from build123d import *

# Parameters (mm, degrees)
F0_R     = 11
F1_DEPTH = 3
F3_DEPTH = 5


with BuildPart() as f1:
    # F0 (on Top) → F1 (new body)
    with BuildSketch(Plane.XY):
        Circle(F0_R)
    extrude(amount=F1_DEPTH)

    # F2 (on face) → F3 (join)
    with BuildSketch(Plane.XY.offset(3)):
        with BuildLine():
            Line((6, 2.5), (6, 4.5))
            ThreePointArc((6, 4.5), (0, 7.5), (-6, 4.5))
            Line((-6, 4.5), (-6, 2.5))
            ThreePointArc((-6, 2.5), (0, 6.5), (6, 2.5))
        make_face()
        with BuildLine():
            Line((6, -4.5), (6, -2.5))
            ThreePointArc((6, -2.5), (0, -6.5), (-6, -2.5))
            Line((-6, -2.5), (-6, -4.5))
            ThreePointArc((-6, -4.5), (0, -7.5), (6, -4.5))
        make_face()
    extrude(amount=F3_DEPTH)


solid = f1.part
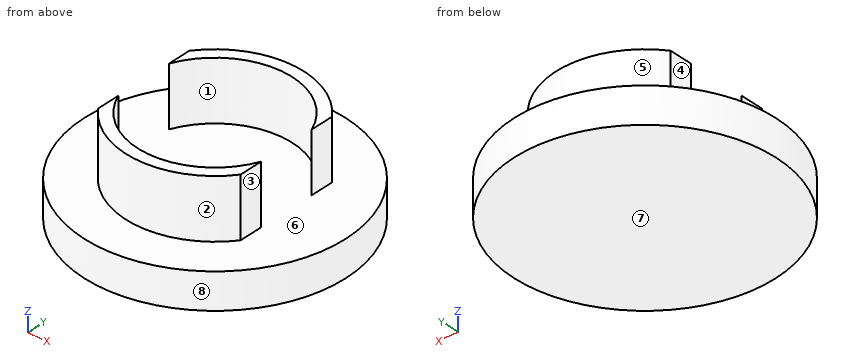
Can you work these out from the model? Positions are in its coordinate system, mm. Face numbers are marked on the shaded views. A direction names the side the tool comes from. Give positions to 0.01 mm unless a question says otherwise; leave off trailing zeros. Loops run counter-clockwise (first coordinate to the right, second up) from the corner with the lowest first, then second, coordinate; pieces in that order, holes last. Notation, with made-up numbers: M 48.5,64 L 88.5,64 A20 cw 88.5,76 Z; hole C 5,81 d10. An arc over 180 degrees is marked long. One line per item, written item: value. Start each with the question number.
1) If we section it at C-C, the plane y = 0: Write out the boundary of the cut face in (x, z), and give its area (3 significant figures).
2) If we section it at B-B, the plane x = 0: Write out the boundary of the cut face in (y, z).
3) If I drill on line 1 (Z direction, x = -2, y = -3.5); line 2 (Y direction, x = 5, z = 6.75); line 3 (Y direction, x = -4.5, z = 5), over which ranges is the centre line in solid material (lowest first)? Write a range as [from, to].
4) On a 3-axis mill with a long thin cutter (end or side, diameter ignored), from which of +Z, -Z, +X, -X, +Y, -Y can I reach the whole of each face in a straight line? I mean the marked faces 1, 2, 3, 4 and 5. Say none if no direction works.
5) If we section it at A-A, the plane z = 5.5: Write out the boundary of the cut face in (x, y).
6) Thinking about a two-plate mould opening in X: for the marked faces 6, 7 and 8, which applies, +X half, -X half, draft (parallel to the pull), parting line (faces both ways), or undercut?
7) If we section it at D-D, the plane z = 1.5: Write out the boundary of the cut face in (x, y), and give its area (3 significant figures).
8) I'm going to push flat-ended pins straight in: pin 1 (1 mm diameter, centred on y = -3, z = 5, fed in from +X); pin 2 (1 mm diameter, centred on y = -3, z = 5.5, fed in from -X); pin 3 (1 mm diameter, centred on x = 2, z = 2, fed in from -Y); pin 4 (10 mm diameter, centred on x = 4, y = -4.5, fed in from +Z). Where does each tip first touch, or does it pass through?
Completed:
1. outline: M -11,0 L 11,0 L 11,3 L -11,3 Z
1. area: 66.0 mm^2
2. outline: M -11,0 L 11,0 L 11,3 L 7.5,3 L 7.5,8 L 6.5,8 L 6.5,3 L -6.5,3 L -6.5,8 L -7.5,8 L -7.5,3 L -11,3 Z
3. line 1: z = [0, 3]
3. line 2: y = [-5.59, -4.15], [4.15, 5.59]
3. line 3: y = [-6, -4.69], [4.69, 6]
4. face 1: +Z
4. face 2: +Z, -Y
4. face 3: +Z, +X, +Y, -Y
4. face 4: +Z, -X, +Y, -Y
4. face 5: +Z, +Y
5. outline: M -6,-4.5 A7.5 ccw 6,-4.5 L 6,-2.5 A6.5 cw -6,-2.5 Z; M -6,2.5 A6.5 cw 6,2.5 L 6,4.5 A7.5 ccw -6,4.5 Z
6. face 6: undercut
6. face 7: draft
6. face 8: parting line
7. outline: C 0,0 d22
7. area: 380 mm^2
8. pin 1: stops at x = 6
8. pin 2: stops at x = -6
8. pin 3: stops at y = -10.9
8. pin 4: stops at z = 8
